from build123d import *

# Parameters (mm, degrees)
F0_R     = 6.35
F1_DEPTH = 7.62
F3_DEPTH = 7.62
F4_R     = 1.5875
F5_DEPTH = 25.4
F6_R     = 2.54


with BuildPart() as f1:
    # F0 (on Top) → F1 (new body)
    with BuildSketch(Plane.XY):
        with BuildLine():
            ThreePointArc((28.575, 0), (25.4, 3.175), (22.225, 0))
            ThreePointArc((22.225, 0), (25.4, -3.175), (28.575, 0))
        make_face()
        Circle(F0_R)
        with BuildLine():
            Line((0, 9.525), (2.344615, 9.231923))
            ThreePointArc((2.344615, 9.231923), (1.181431, 9.451447), (0, 9.525))
        make_face()
        with BuildLine():
            Line((25.4, 6.35), (2.344615, 9.231923))
            Line((2.344615, 9.231923), (0, 9.525))
            ThreePointArc((0, 9.525), (-9.525, 0), (0, -9.525))
            Line((0, -9.525), (2.344615, -9.231923))
            Line((2.344615, -9.231923), (25.4, -6.35))
            ThreePointArc((25.4, -6.35), (31.75, 0), (25.4, 6.35))
        make_face()
        Circle(F0_R, mode=Mode.SUBTRACT)
        with BuildLine():
            ThreePointArc((28.575, 0), (25.4, -3.175), (22.225, 0))
            ThreePointArc((22.225, 0), (25.4, 3.175), (28.575, 0))
        make_face(mode=Mode.SUBTRACT)
        with BuildLine():
            Line((2.344615, -9.231923), (0, -9.525))
            ThreePointArc((0, -9.525), (1.181431, -9.451447), (2.344615, -9.231923))
        make_face()
    extrude(amount=F1_DEPTH)

    # F2 (on face) → F3 (join)
    with BuildSketch(Plane.XY.offset(7.62)):
        Polygon((26.030454, -11.393635), (25.4, -6.35), (2.344615, -9.231923), (3.132236, -15.532888), align=None)
    extrude(amount=-F3_DEPTH)

    # F4 (on face) → F5 (cut)
    with BuildSketch(Plane(origin=(24.227692, 3.028462, 0), x_dir=(-0.124035, 0.992278, 0), z_dir=(0.992278, 0.124035, 0))):
        with Locations((-11.998785, 3.81)):
            Circle(F4_R)
    extrude(amount=-F5_DEPTH, mode=Mode.SUBTRACT)

    # F6
    f6_edges = [f1.edges().sort_by_distance(p)[0] for p in [
        (14.581345, -13.463261, 7.62),
        (14.581345, -13.463261, 0),
    ]]
    fillet(f6_edges, radius=F6_R)


solid = f1.part
Geometry: final body of the model. Coordinates: model frame, mm. Coordinates: 2 decimals unless noted, no trailing zeros. Write each loop counter-clockwise with the first axis right and the second up, starting at its lowest first coordinate (ties: lowest second). Pieces come first, ordered by that corner, then holes. Notation, with made-up numbers: (22.5, 1) - (48.5, 1) arc R35 cw to (48.5, 34) - close; hole circle Ø6 at (-12, 39). An arc over 180 degrees is marked (long way). Return JSON: item names as keys, results as strings.
Item 1: Pin query (flat end, axial travel): pin 1 Ø3 at (x, z) = (-4, 6) entering from -Y. Return the tip coordinate at first contact, or that it passes through.
Completed:
{"pin 1": "stops at y = -9.19"}
Item 2: Line query: L1, parallel to Y at x = 24, z = 2.75 (3 decimals); L2, parallel to Y at x = 3.5, z = 3; L3, parallel to Z at x = 4.5, y = -12.5. Output: solid intervals per line, ascending.
Completed:
{"L1": "y = -11.761 to -10.283, -7.901 to -2.85, 2.85 to 6.525", "L2": "y = -15.47 to -13.03, -10.28 to -5.3, 5.3 to 9.09", "L3": "z = 0 to 2.55, 5.07 to 7.62"}
Item 3: Pull-direction query (Y, two-part tool) for faces 1 (the face through (25.72, -8.91, 5.56)), 2 (the face through (1.2, 9.45, 3.76)), 3 (the face through (14.421, -13.492, 3.828)); classes: +Y half, -Y half, draft (parallel to the pull), parting line (faces both ways), or undercut.
Completed:
{"face 1": "undercut", "face 2": "+Y half", "face 3": "-Y half"}
Item 4: Section query D-D (z = 6.25). Output: boundary loops of the cut face in (x, y) (3 decimals).
Completed:
{"outline": "(0, -9.525) arc R9.525 ccw to (2.345, -9.232) - (3.097, -15.249) - (25.995, -11.11) - (25.4, -6.35) arc R6.35 ccw to (25.4, 6.35) - (2.345, 9.232) arc R9.525 ccw to (0, 9.525) arc R9.525 ccw to start; hole circle Ø12.7 at (0, 0); hole circle Ø6.35 at (25.4, 0)"}
Item 5: Section query A-A (z = 4.5). Output: boundary loops of the cut face in (x, y) (3 decimals), and give its area (3 significant figures).
Completed:
{"outline": "(0, -9.525) arc R9.525 ccw to (2.345, -9.232) - (2.483, -10.341) - (25.539, -7.459) - (25.4, -6.35) arc R6.35 ccw to (25.4, 6.35) - (2.345, 9.232) arc R9.525 ccw to (0, 9.525) arc R9.525 ccw to start; (2.838, -13.178) - (3.132, -15.533) - (26.03, -11.394) - (25.893, -10.296) - close; hole circle Ø12.7 at (0, 0); hole circle Ø6.35 at (25.4, 0)", "area": "517 mm2"}
Item 6: Section query B-B (y = 0). Output: boundary loops of the cut face in (x, z) (3 decimals), and give its area (3 significant figures).
Completed:
{"outline": "(-9.525, 0) - (-6.35, 0) - (-6.35, 7.62) - (-9.525, 7.62) - close; (6.35, 0) - (22.225, 0) - (22.225, 7.62) - (6.35, 7.62) - close; (28.575, 0) - (31.75, 0) - (31.75, 7.62) - (28.575, 7.62) - close", "area": "169 mm2"}
Item 7: Section query C-C (x = -2.5). Output: boundary loops of the cut face in (y, z), and give its area (3 significant figures).
Completed:
{"outline": "(-9.19, 0) - (-5.84, 0) - (-5.84, 7.62) - (-9.19, 7.62) - close; (5.84, 0) - (9.19, 0) - (9.19, 7.62) - (5.84, 7.62) - close", "area": "51.1 mm2"}
